from build123d import *

# Parameters (mm, degrees)
SKETCH_1_R          = 2.05
EXTRUDE_1_DEPTH     = 80
SKETCH_2_W          = 13.5
SKETCH_2_H          = 3.1
CUT_EXTRUDE_1_DEPTH = 95
SKETCH_4_R          = 2.6
CUT_EXTRUDE_2_DEPTH = 20
SKETCH_5_W          = 32.115933716
SKETCH_5_H          = 48
CUT_EXTRUDE_5_DEPTH = 20
FILLET_1_R          = 3


with BuildPart() as part:
    # 草图1 → 凸台-拉伸1 (new body)
    with BuildSketch(Plane.XY):
        with BuildLine():
            Line((0, 5), (21, 5))
            ThreePointArc((21, 5), (26, 0), (21, -5))
            Line((21, -5), (0, -5))
            Line((0, -5), (0, 5))
        make_face()
        with Locations(Location((21, 0, 0), (0, 0, 180))):
            Circle(SKETCH_1_R, mode=Mode.SUBTRACT)
    extrude(amount=EXTRUDE_1_DEPTH)

    # 草图2 → 切除-拉伸1 (cut)
    with BuildSketch(Plane.XY.offset(80)):
        with Locations((6.75, 0)):
            Rectangle(SKETCH_2_W, SKETCH_2_H)
    extrude(amount=-CUT_EXTRUDE_1_DEPTH, mode=Mode.SUBTRACT)

    # 草图4 → 切除-拉伸2 (cut)
    with BuildSketch(Plane(origin=(0, 5, 0), x_dir=(1, 0, 0), z_dir=(0, 1, 0))):
        with Locations((6.5, -32.5)):
            Circle(SKETCH_4_R)
        with Locations((6.5, -7.5)):
            Circle(SKETCH_4_R)
        with Locations((6.5, -72.5)):
            Circle(SKETCH_4_R)
        with Locations((6.5, -47.5)):
            Circle(SKETCH_4_R)
    extrude(amount=-CUT_EXTRUDE_2_DEPTH, mode=Mode.SUBTRACT)

    # 草图5 → 切除-拉伸5 (cut)
    with BuildSketch(Plane(origin=(0, 5, 0), x_dir=(1, 0, 0), z_dir=(0, 1, 0))):
        with Locations((31.057966858, -40)):
            Rectangle(SKETCH_5_W, SKETCH_5_H)
    extrude(amount=-CUT_EXTRUDE_5_DEPTH, mode=Mode.SUBTRACT)

    # 圆角1
    fillet_1_edges = [part.edges().sort_by_distance(p)[0] for p in [
        (0, -3.275, 0),
        (0, -3.275, 80),
        (0, 3.275, 80),
        (0, 3.275, 0),
    ]]
    fillet(fillet_1_edges, radius=FILLET_1_R)


solid = part.part
The listing builds one solid part. Answer for the finished solid, in the listing's coordinates (mm). A direction names the side the tool comes from. Give positions to 0.01 mm unless a question says otherwise; leave off trailing zeros. Write each loop counter-clockwise with the first axis right and the second up, starting at its lowest first coordinate (ties: lowest second). Pieces come first, ordered by that corner, then holes. Notation, with made-up numbers: (83.5, 66) -> (123.5, 66) arc R26 ccw to (123.5, 81) -> close; hole circle Ø9 at (-2, 53.5). An arc over 180 degrees is marked (long way). Use a Markdown table: item, result.
(1) Section C-C, the plane y = 3 is taken. Determine the outline of the cut face in (x, z), then the cut area to 3 significant figures.
Return value:
| item | result |
|---|---|
| outline | (0, 3) arc R3 ccw to (3, 0) -> (25, 0) -> (25, 16) -> (15, 16) -> (15, 64) -> (25, 64) -> (25, 80) -> (3, 80) arc R3 ccw to (0, 77) -> close; hole circle Ø5.2 at (6.5, 7.5); hole circle Ø5.2 at (6.5, 32.5); hole circle Ø5.2 at (6.5, 47.5); hole circle Ø5.2 at (6.5, 72.5) |
| area | 1,430 mm2 |
(2) Section B-B, the plane y = 0 is taken. Determine the outline of the cut face in (x, z).
Return value:
| item | result |
|---|---|
| outline | (13.5, 0) -> (18.95, 0) -> (18.95, 16) -> (15, 16) -> (15, 64) -> (18.95, 64) -> (18.95, 80) -> (13.5, 80) -> close; (23.05, 0) -> (26, 0) -> (26, 16) -> (23.05, 16) -> close; (23.05, 64) -> (26, 64) -> (26, 80) -> (23.05, 80) -> close |
(3) Determine the mould class of faces 4 (the cylindrical face through (0.9, 3.3, 79.14)), 5 (the flat face through (15, 0, 40)), 6 (the cylindrical face through (6.162, 3.299, 29.922)) for opening direction X: released by +X, released by -X, zero draft, split by the parting line, or undercut.
Return value:
| item | result |
|---|---|
| face 4 | released by -X |
| face 5 | released by +X |
| face 6 | undercut |
(4) Flat-ended cylindrical pins translate along their axes: P1, Ø4, axis at x = 6.5, z = 7.5, coming from the +Y side; P2, Ø5.5, axis at x = 21, y = 0, coming from the -Z side; P3, Ø1.6, axis at y = 0, z = 55.5, coming from the -X side; P4, Ø3, axis at y = 1.5, z = 38, coming from the +X side. Find the tip coordinate at first contact, or state that the pin passes through.
Return value:
| item | result |
|---|---|
| P1 | through |
| P2 | z = 0 |
| P3 | x = 13.5 |
| P4 | x = 15 |
(5) For faces 1 (the flat face through (19, -1, 16)), 2 (the flat face through (13.5, 0, 41)), 3 (the cylindrical face through (6.162, -3.251, 69.922)), determine the directions among +Z, -Z, +X, -X, +Y, -Y from which every point of the face is accessible in a straight line to the end or side of a thin tool.
Return value:
| item | result |
|---|---|
| face 1 | +X, +Y, -Y |
| face 2 | +Z, -Z, -X |
| face 3 | +Y, -Y |
(6) Find the intervals of material crossed by probe 1 along Z at (x, y) = (6.5, 3.55); probe 2 along X at (y, z) = (3.9, 47.5); probe 3 along Y at (x, z) = (21, 71.5), in increasing order. Write a range as from..to.
Return value:
| item | result |
|---|---|
| probe 1 | 0..4.9, 10.1..29.9, 35.1..44.9, 50.1..69.9, 75.1..80 |
| probe 2 | 0..3.9, 9.1..15 |
| probe 3 | -5..-2.05, 2.05..5 |
(7) Section A-A, the plane z = 47.5 is taken. Determine the outline of the cut face in (x, y).
Return value:
| item | result |
|---|---|
| outline | (0, -5) -> (3.9, -5) -> (3.9, -1.55) -> (0, -1.55) -> close; (0, 1.55) -> (3.9, 1.55) -> (3.9, 5) -> (0, 5) -> close; (9.1, -5) -> (15, -5) -> (15, 5) -> (9.1, 5) -> (9.1, 1.55) -> (13.5, 1.55) -> (13.5, -1.55) -> (9.1, -1.55) -> close |
(8) Section D-D, the plane z = 7.5 is taken. Determine the outline of the cut face in (x, y).
Return value:
| item | result |
|---|---|
| outline | (0, -5) -> (3.9, -5) -> (3.9, -1.55) -> (0, -1.55) -> close; (0, 1.55) -> (3.9, 1.55) -> (3.9, 5) -> (0, 5) -> close; (9.1, -5) -> (21, -5) arc R5 ccw to (21, 5) -> (9.1, 5) -> (9.1, 1.55) -> (13.5, 1.55) -> (13.5, -1.55) -> (9.1, -1.55) -> close; hole circle Ø4.1 at (21, 0) |
